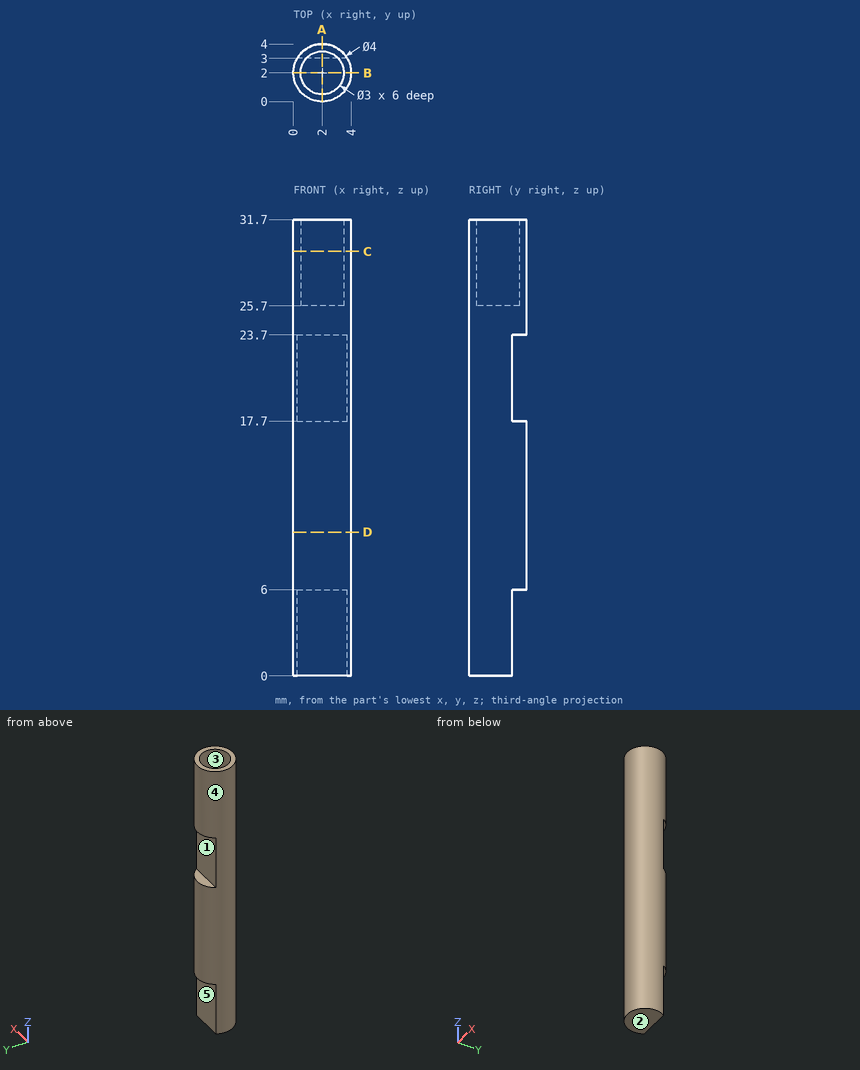
Geometry check sheet. Reference: drawing and pictorial views, mm from the part's lowest x, y, z. A direction names the side the tool comes from. Give positions to 0.01 mm unless a question says otherwise; leave off trailing zeros. Write each loop counter-clockwise with the first axis right and the second up, starting at its lowest first coordinate (ties: lowest second). Pieces come first, ordered by that corner, then holes. Notation, with made-up numbers: (45, 80) -> (86, 80) arc R5 cw to (86, 85) -> close; hole circle Ø6 at (50, -14.5). An arc over 180 degrees is marked (long way). One line per item, written item: value. Start each with the question number.
Item 1: Section check B-B on y = 2. Record the cut outline in (x, z).
Item 2: Section check C-C on z = 29.5. Record the cut outline in (x, y), then the cut area to 3 significant figures.
Item 3: Gauge pin test, flat ends, axial feed: pin 1 (1.1 mm diameter, centred on x = 3, y = 3.5, fed in from -Z); pin 2 (1 mm diameter, centred on x = 1.5, z = 22, fed in from +Y); pin 3 (1.5 mm diameter, centred on x = 2.5, y = 1.5, fed in from +Z); pin 4 (0.5 mm diameter, centred on x = 2, y = 3.5, fed in from -Z). Record the tip position at first contact, or that the pin passes through.
Item 4: Section check D-D on z = 10. Record the cut outline in (x, y), then the cut area to 3 significant figures.
Item 5: Section check A-A on x = 2. Record the cut outline in (y, z).
Item 6: Draft check along Y on the marked faces 3, 4 and 5. Enter one of: +Y half, -Y half, draft (parallel to the pull), parting line (faces both ways), or undercut.
Item 7: Tool access check on the marked faces 1 and 2. Record the directions out of +Z, -Z, +X, -X, +Y, -Y that give a thin tool (end or side, any length) a straight path to the whole face; none if there is none.
Item 8: Material ranges on probe 1 along X at (y, z) = (2, 28.25); probe 2 along Z at (x, y) = (2.5, 3.55); probe 3 along Z at (x, y) = (1.2, 1.8), recorded low to high. Write a range as from..to.
Results list:
1. outline: (0, 0) -> (4, 0) -> (4, 31.7) -> (3.5, 31.7) -> (3.5, 25.7) -> (0.5, 25.7) -> (0.5, 31.7) -> (0, 31.7) -> close
2. outline: circle Ø4 at (2, 2); hole circle Ø3 at (2, 2)
2. area: 5.50 mm²
3. pin 1: z = 0
3. pin 2: y = 3
3. pin 3: z = 25.7
3. pin 4: z = 6
4. outline: circle Ø4 at (2, 2)
4. area: 12.6 mm²
5. outline: (0, 0) -> (3, 0) -> (3, 6) -> (4, 6) -> (4, 17.7) -> (3, 17.7) -> (3, 23.7) -> (4, 23.7) -> (4, 31.7) -> (3.5, 31.7) -> (3.5, 25.7) -> (0.5, 25.7) -> (0.5, 31.7) -> (0, 31.7) -> close
6. face 3: undercut
6. face 4: parting line
6. face 5: +Y half
7. face 1: +X, -X, +Y
7. face 2: -Z, +X, -X, +Y, -Y
8. probe 1: 0..0.5, 3.5..4
8. probe 2: 6..17.7, 23.7..31.7
8. probe 3: 0..25.7
